Design review of the part built by this model. Coordinates are the model's own, in mm. Give positions to 0.01 mm unless a question says otherwise; leave off trailing zeros. Write each loop counter-clockwise with the first axis right and the second up, starting at its lowest first coordinate (ties: lowest second). Pieces come first, ordered by that corner, then holes.
```python
from build123d import *

# Parameters (mm, degrees)
SKETCH_1_R          = 1.65
EXTRUDE_1_DEPTH     = 3
SKETCH_2_R          = 1.65
CUT_EXTRUDE_1_DEPTH = 109.673823895


with BuildPart() as part:
    # Эскиз1 → Бобышка-Вытянуть1 (new body)
    with BuildSketch(Plane.XY):
        with BuildLine():
            Line((-34, 101), (34, 101))
            ThreePointArc((34, 101), (38.242640687, 99.242640687), (40, 95))
            Line((40, 95), (40, -95))
            ThreePointArc((40, -95), (38.242640687, -99.242640687), (34, -101))
            Line((34, -101), (-34, -101))
            ThreePointArc((-34, -101), (-38.242640687, -99.242640687), (-40, -95))
            Line((-40, -95), (-40, 95))
            ThreePointArc((-40, 95), (-38.242640687, 99.242640687), (-34, 101))
        make_face()
        with Locations((-35, 91)):
            Circle(SKETCH_1_R, mode=Mode.SUBTRACT)
        with Locations((-35, 35)):
            Circle(SKETCH_1_R, mode=Mode.SUBTRACT)
        with Locations(Location((35, 35, 0), (0, 0, 180))):
            Circle(SKETCH_1_R, mode=Mode.SUBTRACT)
        with Locations(Location((35, 91, 0), (0, 0, 180))):
            Circle(SKETCH_1_R, mode=Mode.SUBTRACT)
        with Locations((35, -91)):
            Circle(SKETCH_1_R, mode=Mode.SUBTRACT)
        with Locations(Location((-35, -91, 0), (0, 0, 180))):
            Circle(SKETCH_1_R, mode=Mode.SUBTRACT)
        with Locations(Location((-35, -35, 0), (0, 0, 180))):
            Circle(SKETCH_1_R, mode=Mode.SUBTRACT)
        with Locations((35, -35)):
            Circle(SKETCH_1_R, mode=Mode.SUBTRACT)
    extrude(amount=EXTRUDE_1_DEPTH)

    # Эскиз2 → Вырез-Вытянуть1 (cut, through all)
    with BuildSketch(Plane.XY.offset(3)):
        with Locations((-26.25, -88.75)):
            Circle(SKETCH_2_R)
        with Locations((26.25, -88.75)):
            Circle(SKETCH_2_R)
        with BuildLine():
            Line((-22, 25), (-22, -25))
            ThreePointArc((-22, -25), (-23.5, -26.5), (-25, -25))
            Line((-25, -25), (-25, 25))
            ThreePointArc((-25, 25), (-23.5, 26.5), (-22, 25))
        make_face()
        with BuildLine():
            Line((22, 25), (22, -25))
            ThreePointArc((22, -25), (23.5, -26.5), (25, -25))
            Line((25, -25), (25, 25))
            ThreePointArc((25, 25), (23.5, 26.5), (22, 25))
        make_face()
        with BuildLine():
            Line((-23.5, -75), (23.5, -75))
            ThreePointArc((23.5, -75), (25, -73.5), (23.5, -72))
            Line((23.5, -72), (-23.5, -72))
            ThreePointArc((-23.5, -72), (-25, -73.5), (-23.5, -75))
        make_face()
    extrude(amount=-CUT_EXTRUDE_1_DEPTH, mode=Mode.SUBTRACT)


solid = part.part
```
(1) To check wall thickness, follow L1, parallel to X at y = -2, z = 1.9; L2, parallel to X at y = 91, z = 1.65; L3, parallel to Y at x = 3, z = 1.5. State the ranges of each line that lie inside material, in increasing order.
Resolved:
L1: x = -40 to -25, -22 to 22, 25 to 40
L2: x = -40 to -36.65, -33.35 to 33.35, 36.65 to 40
L3: y = -101 to -75, -72 to 101
(2) Consider section A-A, the plane y = 8.5. Give the boundary of the cut face in (x, z), then the cut area to 3 significant figures.
Resolved:
outline: (-40, 0) - (-25, 0) - (-25, 3) - (-40, 3) - close; (-22, 0) - (22, 0) - (22, 3) - (-22, 3) - close; (25, 0) - (40, 0) - (40, 3) - (25, 3) - close
area: 222 mm2
(3) Consider section B-B, the plane z = 1.1. Give the number of separate pieces and of enclosed holes in the cut face, then the cut area to 3 significant figures.
Resolved:
separate pieces: 1
enclosed holes: 13
area: 15,600 mm2
(4) Mouldability with a two-part tool opening along Y and no side actions: class faces 1 (the face through (-33.784, -36.115, 1.479)), 2 (the face through (38.196, 99.289, 1.479)), 3 (the face through (38.289, -99.196, 1.479)), 4 (the face through (35.4, 92.6, 1.5)) as pulls with the +Y half, pulls with the -Y half, needs draft (parallel to the pull), parting line crosses it, or undercut.
Resolved:
face 1: undercut
face 2: pulls with the +Y half
face 3: pulls with the -Y half
face 4: undercut
(5) Clearance check with a flat-ended pin moving along its axis: P1, Ø3, axis at x = -35, y = 35, coming from the -Z side. State where the tip first meets the part, or that it passes through.
Resolved:
P1: passes through
